Read the model definition and answer for the solid it produces. Units are mm, in the model's axes. Give positions to 0.01 mm unless a question says otherwise; leave off trailing zeros. Loops run counter-clockwise (first coordinate to the right, second up) from the corner with the lowest first, then second, coordinate; pieces in that order, holes last. Notation, with made-up numbers: (-9.5, -27.75) -> (3.5, -27.75) arc R20 cw to (3.5, -7.75) -> close; hole circle Ø4 at (41.5, 29.25). An arc over 180 degrees is marked (long way). One line per item, written item: value. Start each with the question number.
Autodesk Inventor part; units mm, degrees
ref_plane "YZ Plane" through (0, 0, 0) normal (1, 0, 0) x (0, 1, 0)
ref_plane "XZ Plane" through (0, 0, 0) normal (0, 1, 0) x (-1, 0, 0)
ref_plane "XY Plane" through (0, 0, 0) normal (0, 0, 1) x (1, 0, 0)
sketch "Sketch1" plane through (0, 0, 0) normal (0, 0, 1) x (1, 0, 0)
  line L0 (0, 0) -> (20, 0)
  line L1 (20, 0) -> (20, 30)
  line L2 (20, 30) -> (0, 30)
  line L3 (0, 30) -> (0, 0)
  dimension "d0" = 20
  dimension "d1" = 30
extrude "Extrusion1" add sketch "Sketch1" along normal blind 3
sketch "Sketch2" plane through (0, 0, 3) normal (0, 0, 1) x (1, 0, 0)
  line L0 (0, 0) -> (20, 0)
  line L1 (20, 0) -> (20, 30)
  line L2 (20, 30) -> (0, 30)
  line L3 (0, 30) -> (0, 0)
  line L4 (0, 5) -> (20, 5)
  line L5 (10, 0) -> (10, 30)
  circle A0 centre (5, 5) radius 1.5
  circle A1 centre (15, 5) radius 1.5
  dimension "d4" = 3
  dimension "d5" = 10
  dimension "d6" = 10
extrude "Extrusion2" cut sketch "Sketch2" against normal blind 3 contours A0 L4 | L4 A0 | A1 L4 | L4 A1
sketch "Sketch4" plane through (0, 0, 3) normal (0, 0, 1) x (1, 0, 0)
  line L0 (0, 0) -> (20, 0)
  line L1 (20, 30) -> (0, 30)
  line L2 (10, 30) -> (10, 0)
  circle A0 centre (10, 20.5) radius 1.5
  dimension "d13" = 3
  dimension "d14" = 9.5
extrude "Extrusion4" cut sketch "Sketch4" against normal blind 3
properties part number "limit-holders"
Item 1: Section C-C, the plane y = 5 is taken. Determine the outline of the cut face in (x, z).
Item 2: Determine the mould class of faces 1 (the flat face through (10, 30, 1)), 2 (the cylindrical face through (13.5, 5.07, 1.52)), 3 (the flat face through (10, 0, 1)) for opening direction Y: pulls with the +Y half, pulls with the -Y half, needs draft (parallel to the pull), parting line crosses it, or undercut.
Item 3: Section B-B, the plane x = 4.5 is taken. Determine the outline of the cut face in (y, z).
Item 4: Section A-A, the plane y = 20.5 is taken. Determine the outline of the cut face in (x, z), plus the area to 3 significant figures.
Item 5: Section D-D, the plane z = 0.7 is taken. Determine the outline of the cut face in (x, y), plus the area to 3 significant figures.
Item 6: Consider L1, parallel to X at y = 5, z = 1.4; L2, parallel to Y at x = 10, z = 0.6; L3, parallel to Y at x = 5, z = 2. Determine where each line is inside the solid, lowest interval first. Write a range as [from, to].
Computed values:
1. outline: (0, 0) -> (3.5, 0) -> (3.5, 3) -> (0, 3) -> close; (6.5, 0) -> (13.5, 0) -> (13.5, 3) -> (6.5, 3) -> close; (16.5, 0) -> (20, 0) -> (20, 3) -> (16.5, 3) -> close
2. face 1: pulls with the +Y half
2. face 2: undercut
2. face 3: pulls with the -Y half
3. outline: (0, 0) -> (3.59, 0) -> (3.59, 3) -> (0, 3) -> close; (6.41, 0) -> (30, 0) -> (30, 3) -> (6.41, 3) -> close
4. outline: (0, 0) -> (8.5, 0) -> (8.5, 3) -> (0, 3) -> close; (11.5, 0) -> (20, 0) -> (20, 3) -> (11.5, 3) -> close
4. area: 51.0 mm²
5. outline: (0, 0) -> (20, 0) -> (20, 30) -> (0, 30) -> close; hole circle Ø3 at (5, 5); hole circle Ø3 at (10, 20.5); hole circle Ø3 at (15, 5)
5. area: 579 mm²
6. L1: [0, 3.5], [6.5, 13.5], [16.5, 20]
6. L2: [0, 19], [22, 30]
6. L3: [0, 3.5], [6.5, 30]
